Read the model definition and answer for the solid it produces. Units are mm, in the model's axes. Give positions to 0.01 mm unless a question says otherwise; leave off trailing zeros. Write each loop counter-clockwise with the first axis right and the second up, starting at its lowest first coordinate (ties: lowest second). Pieces come first, ordered by that corner, then holes. Notation, with made-up numbers: (13.5, 62.25) -> (28.5, 62.25) arc R20 ccw to (28.5, 68.25) -> close; hole circle Ø3 at (-5, -20.5). An arc over 180 degrees is marked (long way). Put each result on its own line as item: value. Start each with the question number.
from build123d import *

# Parameters (mm, degrees)
SKETCH_4_W      = 60
SKETCH_4_H      = 115
EXTRUDE_1_DEPTH = 2
SKETCH_5_W      = 8.571428572
SKETCH_5_H      = 2
EXTRUDE_2_DEPTH = 4.5
EXTRUDE_START   = -115
SKETCH_5_3_W    = 8.571428572
SKETCH_5_3_H    = 2
EXTRUDE_3_DEPTH = 4.3
SKETCH_6_W      = 16.428571428
SKETCH_6_H      = 2
EXTRUDE_4_DEPTH = 2
EXTRUDE_START_2 = -60
SKETCH_6_2_W    = 16.428571428
SKETCH_6_2_H    = 2
EXTRUDE_5_DEPTH = 2


with BuildPart() as part:
    # 草图4 → 凸台-拉伸1 (new body)
    with BuildSketch(Plane(origin=(0, 0, 0), x_dir=(1, 0, 0), z_dir=(0, 1, 0))):
        Rectangle(SKETCH_4_W, SKETCH_4_H)
    extrude(amount=EXTRUDE_1_DEPTH)

    # 草图5 → 凸台-拉伸2 (add)
    with BuildSketch(Plane.XY.offset(57.5)):
        with Locations((17.142857143, 1)):
            Rectangle(SKETCH_5_W, SKETCH_5_H)
        with Locations((0, 1)):
            Rectangle(SKETCH_5_W, SKETCH_5_H)
        with Locations((-17.142857143, 1)):
            Rectangle(SKETCH_5_W, SKETCH_5_H)
    extrude(amount=EXTRUDE_2_DEPTH)

    # 草图5<3> → 凸台-拉伸3 (add)
    with BuildSketch(Plane.XY.offset(57.5).offset(EXTRUDE_START)):
        with Locations((17.142857143, 1)):
            Rectangle(SKETCH_5_3_W, SKETCH_5_3_H)
        with Locations((0, 1)):
            Rectangle(SKETCH_5_3_W, SKETCH_5_3_H)
        with Locations((-17.142857143, 1)):
            Rectangle(SKETCH_5_3_W, SKETCH_5_3_H)
    extrude(amount=-EXTRUDE_3_DEPTH)

    # 草图6 → 凸台-拉伸4 (add)
    with BuildSketch(Plane(origin=(30, 0, 0), x_dir=(0, 0, -1), z_dir=(1, 0, 0))):
        with Locations((-32.857142857, 1)):
            Rectangle(SKETCH_6_W, SKETCH_6_H)
        with Locations((0, 1)):
            Rectangle(SKETCH_6_W, SKETCH_6_H)
        with Locations((32.857142857, 1)):
            Rectangle(SKETCH_6_W, SKETCH_6_H)
    extrude(amount=EXTRUDE_4_DEPTH)

    # 草图6<2> → 凸台-拉伸5 (add)
    with BuildSketch(Plane(origin=(30, 0, 0), x_dir=(0, 0, -1), z_dir=(1, 0, 0)).offset(EXTRUDE_START_2)):
        with Locations((-32.857142857, 1)):
            Rectangle(SKETCH_6_2_W, SKETCH_6_2_H)
        with Locations((0, 1)):
            Rectangle(SKETCH_6_2_W, SKETCH_6_2_H)
        with Locations((32.857142857, 1)):
            Rectangle(SKETCH_6_2_W, SKETCH_6_2_H)
    extrude(amount=-EXTRUDE_5_DEPTH)


solid = part.part
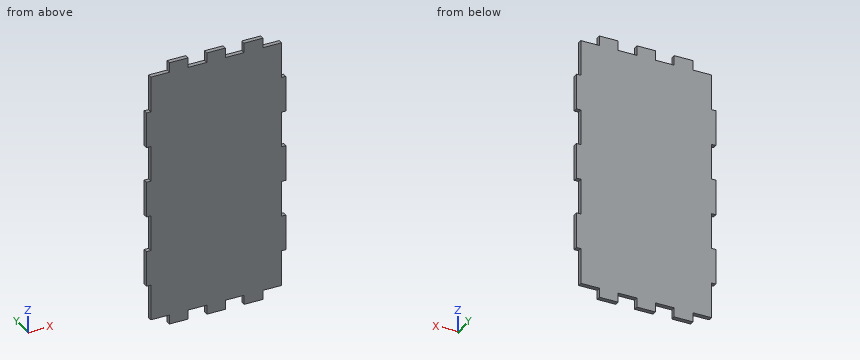
1) Straight lines are drawn through the part: line 1 (Z direction, x = 8, y = 1.6); line 2 (X direction, y = 1, z = -50.5). For each, find the intervals that lie inside material, in ascending order. Write a range as [from, to].
2) A cutting plane is placed at A-A on x = 25. Give the vertices of the cut face in (y, z).
3) A cutting plane is placed at B-B on z = -10. Give the vertices of the cut face in (x, y).
4) Each of these flat-tipped pins is pushed along its axis until it touches: pin 1 Ø6 at (x, z) = (-15.5, -2) entering from -Y; pin 2 Ø1 at (y, z) = (1, -60.5) entering from +X; pin 3 Ø0.6 at (y, z) = (1, -20) entering from -X; pin 4 Ø0.6 at (x, y) = (31, 0.5) entering from +Z. Where does it stop, or does it pass through?
Results found:
1. line 1: z = [-57.5, 57.5]
1. line 2: x = [-30, 30]
2. outline: (0, -57.5) -> (2, -57.5) -> (2, 57.5) -> (0, 57.5) -> close
3. outline: (-30, 0) -> (30, 0) -> (30, 2) -> (-30, 2) -> close
4. pin 1: stops at y = 0
4. pin 2: stops at x = 21.43
4. pin 3: stops at x = -30
4. pin 4: stops at z = 41.07
